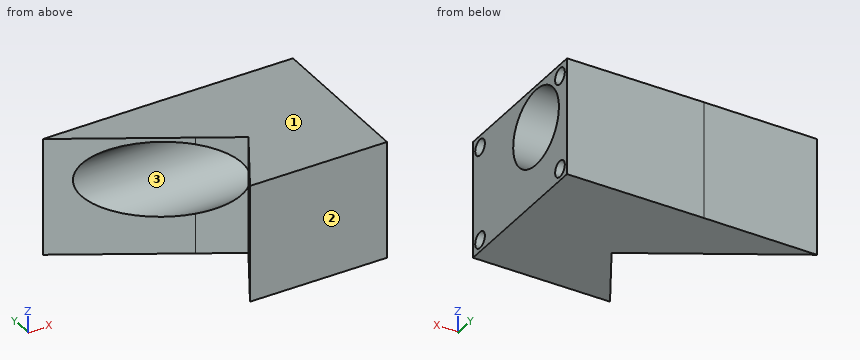
from build123d import *

# Parameters (mm, degrees)
SKETCH2_W                       = 44.45
SKETCH2_H                       = 50.8
BOSS_EXTRUDE2_DEPTH             = 38.1
F_5_0_2055_DIAMETER_HOLE1_D     = 5.2197
F_5_0_2055_DIAMETER_HOLE1_DEPTH = 12.7
F_5_0_2055_DIAMETER_HOLE1_TIP   = 1.568156087
BOSS_EXTRUDE3_DEPTH             = 38.1
CUT_EXTRUDE2_DEPTH              = 39.1
SKETCH3_R                       = 12.342015131
CUT_EXTRUDE1_DEPTH              = 1
CUT_EXTRUDE1_DEPTH_BACK         = 82.243351826


with BuildPart() as part:
    # Sketch2 → Boss-Extrude2 (new body)
    with BuildSketch(Plane.XY):
        with Locations((-18.295089844, 0.954798727)):
            Rectangle(SKETCH2_W, SKETCH2_H)
    extrude(amount=BOSS_EXTRUDE2_DEPTH)

    # #5 (0.2055) Diameter Hole1
    with Locations(Plane(origin=(3.929910156, 22.544798727, 34.29), x_dir=(0, 1, 0), z_dir=(1, 0, 0))):
        with Locations((0, 0), (0, -30.48), (-43.18, -30.48), (-43.18, 0)):
            Hole(F_5_0_2055_DIAMETER_HOLE1_D / 2, depth=F_5_0_2055_DIAMETER_HOLE1_DEPTH)
            with Locations((0, 0, -(F_5_0_2055_DIAMETER_HOLE1_DEPTH + F_5_0_2055_DIAMETER_HOLE1_TIP / 2))):  # 118° drill point
                Cone(0, F_5_0_2055_DIAMETER_HOLE1_D / 2, F_5_0_2055_DIAMETER_HOLE1_TIP, mode=Mode.SUBTRACT)

    # Sketch6 → Boss-Extrude3 (add)
    with BuildSketch(Plane(origin=(0, 0, 0), x_dir=(-1, 0, 0), z_dir=(0, 0, -1))):
        Polygon((40.520089844, 26.354798727), (77.31344167, 26.126843983), (40.520089844, 4.884192402), align=None)
    extrude(amount=-BOSS_EXTRUDE3_DEPTH)

    # Sketch7 → Cut-Extrude2 (cut, through all)
    with BuildSketch(Plane(origin=(0, 0, 0), x_dir=(-1, 0, 0), z_dir=(0, 0, -1))):
        Polygon((40.520089844, 4.884192402), (27.820089844, -2.448156017), (40.520089844, -24.445201273), align=None)
    extrude(amount=-CUT_EXTRUDE2_DEPTH, mode=Mode.SUBTRACT)

    # Sketch3 → Cut-Extrude1 (cut, two sides)
    with BuildSketch(Plane(origin=(3.929910156, 0, 0), x_dir=(0, 0, -1), z_dir=(1, 0, 0))) as cut_extrude1_sk:
        with Locations((-24.476370381, 9.6189509)):
            Circle(SKETCH3_R)
    extrude(amount=CUT_EXTRUDE1_DEPTH, mode=Mode.SUBTRACT)
    extrude(cut_extrude1_sk.sketch, amount=-CUT_EXTRUDE1_DEPTH_BACK, mode=Mode.SUBTRACT)


solid = part.part
Input: part model. Units: mm. Frame: model coordinates. Face numbers are marked on the shaded views. Round coordinates to 2 decimals unless told otherwise and drop trailing zeros. Order: outer loops, then holes, each group sorted by start corner. A loop starts at its lowest first (then second) coordinate and runs counter-clockwise, first axis right, second up. Notation, with made-up numbers: (-3, 84.5) - (50, 84.5) arc R26 ccw to (50, 109.5) - close; hole circle Ø1 at (75, -13.5). An arc over 180 degrees is marked (long way). Use a Markdown table: item, result.
1. Material intervals for probe 1 along Z at (x, y) = (-2, 9); probe 2 along Y at (x, z) = (0, 3); probe 3 along Y at (x, z) = (-4.75, 34.29), sorted ascending.
Evaluation:
| item | result |
|---|---|
| probe 1 | 0 to 12.15, 36.8 to 38.1 |
| probe 2 | -24.45 to -23.12, -18.15 to 20.06, 25.03 to 26.35 |
| probe 3 | -24.45 to -23.25, -18.03 to 2.13, 17.1 to 19.93, 25.15 to 26.35 |
2. First-contact query: pin 1 (3 mm diameter, centred on x = -23, y = -15.5, fed in from -Z); pin 2 (4 mm diameter, centred on y = -20.64, z = 3.81, fed in from +X); pin 3 (15 mm diameter, centred on y = 9.62, z = 24.48, fed in from +X); pin 4 (5 mm diameter, centred on x = -62, z = 32.5, fed in from +Y). Flat tips, straight axial feed; report the tip coordinate or a pass-through.
Evaluation:
| item | result |
|---|---|
| pin 1 | z = 0 |
| pin 2 | x = -9.13 |
| pin 3 | through |
| pin 4 | y = 26.24 |
3. Section C-C on x = -6.5. Return the cut outline in (y, z).
Evaluation:
| item | result |
|---|---|
| outline | (-24.45, 0) - (26.35, 0) - (26.35, 38.1) - (-24.45, 38.1) - close; hole circle Ø5.22 at (-20.64, 3.81); hole circle Ø5.22 at (-20.64, 34.29); hole circle Ø24.68 at (9.62, 24.48); hole circle Ø5.22 at (22.54, 3.81); hole circle Ø5.22 at (22.54, 34.29) |
4. Mould query, pull axis Z, two halves, no side actions, for the marked faces 1, 2 and 3. Classes: +Z half, -Z half, draft (parallel to the pull), parting line (faces both ways), or undercut.
Evaluation:
| item | result |
|---|---|
| face 1 | +Z half |
| face 2 | draft |
| face 3 | undercut |
5. Section A-A on x = -30.5. Return the cut outline in (y, z), then the cut area to 3 significant figures.
Evaluation:
| item | result |
|---|---|
| outline | (-24.45, 0) - (-7.09, 0) - (-7.09, 38.1) - (-24.45, 38.1) - close; (-0.9, 0) - (26.35, 0) - (26.35, 38.1) - (-0.9, 38.1) - (-0.9, 30.93) arc R12.34 cw (long way) to (-0.9, 18.02) - close |
| area | 1,240 mm^2 |
6. Section D-D on z = 16. Return the cut outline in (x, y), then the cut area to 3 significant figures.
Evaluation:
| item | result |
|---|---|
| outline | (-77.31, 26.13) - (-64.26, 18.59) - (3.93, 18.59) - (3.93, 26.35) - (-40.52, 26.35) - close; (-40.52, -24.45) - (3.93, -24.45) - (3.93, 0.65) - (-33.18, 0.65) - (-27.82, -2.45) - close |
| area | 1,520 mm^2 |
7. Section B-B on y = 7. Return the cut outline in (x, z).
Evaluation:
| item | result |
|---|---|
| outline | (-44.18, 0) - (3.93, 0) - (3.93, 12.42) - (-44.18, 12.42) - close; (-44.18, 36.54) - (3.93, 36.54) - (3.93, 38.1) - (-44.18, 38.1) - close |
